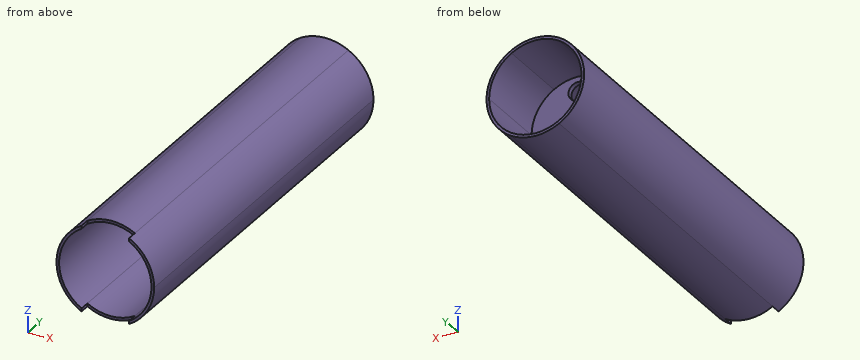
```python
from build123d import *

# Parameters (mm, degrees)
SHELL_DEPTH        = 150
SKETCH8_R          = 17.5
SKETCH8_R_2        = 3.5
SKETCH8_R_3        = 6.5
RODALIGNER_DEPTH   = 1
CUT_EXTRUDE1_DEPTH = 4


with BuildPart() as part:
    # Sketch1 → Shell (new body)
    with BuildSketch(Plane(origin=(0, 0, 0), x_dir=(1, 0, 0), z_dir=(0, 1, 0))):
        with BuildLine():
            ThreePointArc((-9.013878189, -15), (-17.5, 0), (-9.013878189, 15))
            Line((-9.013878189, 15), (-9.013878189, 16.155494421))
            ThreePointArc((-9.013878189, 16.155494421), (-18.5, 0), (-9.013878189, -16.155494421))
            Line((-9.013878189, -16.155494421), (-9.013878189, -15))
        make_face()
        with BuildLine():
            ThreePointArc((9.013878189, -15), (0, -17.5), (-9.013878189, -15))
            Line((-9.013878189, -15), (-9.013878189, -16.155494421))
            ThreePointArc((-9.013878189, -16.155494421), (0, -18.5), (9.013878189, -16.155494421))
            Line((9.013878189, -16.155494421), (9.013878189, -15))
        make_face()
        with BuildLine():
            Line((-9.013878189, 16.155494421), (-9.013878189, 15))
            ThreePointArc((-9.013878189, 15), (0, 17.5), (9.013878189, 15))
            Line((9.013878189, 15), (9.013878189, 16.155494421))
            ThreePointArc((9.013878189, 16.155494421), (0, 18.5), (-9.013878189, 16.155494421))
        make_face()
        with BuildLine():
            Line((9.013878189, 16.155494421), (9.013878189, 15))
            ThreePointArc((9.013878189, 15), (15.231429157, 8.617050879), (17.5, 0))
            ThreePointArc((17.5, 0), (15.231429157, -8.617050879), (9.013878189, -15))
            Line((9.013878189, -15), (9.013878189, -16.155494421))
            ThreePointArc((9.013878189, -16.155494421), (15.953161857, -9.367316945), (18.5, 0))
            ThreePointArc((18.5, 0), (15.953161857, 9.367316945), (9.013878189, 16.155494421))
        make_face()
    extrude(amount=SHELL_DEPTH)

    # Sketch8 → RodAligner (add, symmetric)
    with BuildSketch(Plane(origin=(0, 120, 0), x_dir=(1, 0, 0), z_dir=(0, 1, 0))):
        Circle(SKETCH8_R)
        with Locations((0, -12)):
            Circle(SKETCH8_R_2, mode=Mode.SUBTRACT)
        Circle(SKETCH8_R_3, mode=Mode.SUBTRACT)
    extrude(amount=RODALIGNER_DEPTH, both=True)

    # Sketch1_7 → Cut-Extrude1 (cut)
    with BuildSketch(Plane(origin=(0, 0, 0), x_dir=(1, 0, 0), z_dir=(0, 1, 0))):
        with BuildLine():
            Line((-9.013878189, 16.155494421), (-9.013878189, 15))
            ThreePointArc((-9.013878189, 15), (0, 17.5), (9.013878189, 15))
            Line((9.013878189, 15), (9.013878189, 16.155494421))
            ThreePointArc((9.013878189, 16.155494421), (0, 18.5), (-9.013878189, 16.155494421))
        make_face()
        with BuildLine():
            ThreePointArc((9.013878189, -15), (0, -17.5), (-9.013878189, -15))
            Line((-9.013878189, -15), (-9.013878189, -16.155494421))
            ThreePointArc((-9.013878189, -16.155494421), (0, -18.5), (9.013878189, -16.155494421))
            Line((9.013878189, -16.155494421), (9.013878189, -15))
        make_face()
    extrude(amount=CUT_EXTRUDE1_DEPTH, mode=Mode.SUBTRACT)


solid = part.part
```
Can you work these out from the model? Positions are in its coordinate system, mm. Coordinates: 2 decimals unless noted, no trailing zeros. Loops run counter-clockwise (first coordinate to the right, second up) from the corner with the lowest first, then second, coordinate; pieces in that order, holes last. Notation, with made-up numbers: (31.5, 14) -> (65.5, 14) arc R32 ccw to (65.5, 52) -> close; hole circle Ø11 at (-22, 6). An arc over 180 degrees is marked (long way). Put each result on its own line as item: value. Start each with the question number.
Q1. I want a section at A-A (x = 0). Write out the boundary of the cut face in (y, z), plus the area to 3 significant figures.
Q2. I want a section at C-C (z = 12). Write out the boundary of the cut face in (x, y).
Q3. I want a section at B-B (y = 10). Write out the boundary of the cut face in (x, z), plus the area to 3 significant figures.
Q4. If I drill on line 1 (Z direction, x = 0.5, y = 38); line 2 (Y direction, x = 9, z = -0.5); line 3 (X direction, y = 33, z = 9), over which ranges is the centre line in solid material (lowest first)? Write a range as [from, to].
Q5. I want a section at D-D (x = -16). Write out the boundary of the cut face in (y, z).
Q6. I'm going to push flat-ended pins straight in: P1, Ø17.5, axis at x = 0.5, z = 3, coming from the +Y side; P2, Ø1.1, axis at x = 1, z = -16.5, coming from the -Y side; P3, Ø8, axis at y = 132.5, z = -14, coming from the +X side; P4, Ø12, axis at x = -12, z = 3.5, coming from the +Y side. Where does each tip first touch, or does it pass through?
Taken from the geometry:
1. outline: (4, -18.5) -> (150, -18.5) -> (150, -17.5) -> (121, -17.5) -> (121, -6.5) -> (119, -6.5) -> (119, -17.5) -> (4, -17.5) -> close; (4, 17.5) -> (119, 17.5) -> (119, 15.5) -> (121, 15.5) -> (121, 17.5) -> (150, 17.5) -> (150, 18.5) -> (4, 18.5) -> close; (119, 6.5) -> (121, 6.5) -> (121, 8.5) -> (119, 8.5) -> close
1. area: 322 mm2
2. outline: (-14.08, 0) -> (-12.74, 0) -> (-12.74, 119) -> (-3.5, 119) -> (-3.5, 121) -> (-12.74, 121) -> (-12.74, 150) -> (-14.08, 150) -> close; (3.5, 119) -> (12.74, 119) -> (12.74, 0) -> (14.08, 0) -> (14.08, 150) -> (12.74, 150) -> (12.74, 121) -> (3.5, 121) -> close
3. outline: circle Ø37 at (0, 0); hole circle Ø35 at (0, 0)
3. area: 113 mm2
4. line 1: z = [-18.49, -17.49], [17.49, 18.49]
4. line 2: y = [119, 121]
4. line 3: x = [-16.16, -15.01], [15.01, 16.16]
5. outline: (0, -9.29) -> (150, -9.29) -> (150, -7.09) -> (121, -7.09) -> (121, 7.09) -> (150, 7.09) -> (150, 9.29) -> (0, 9.29) -> (0, 7.09) -> (119, 7.09) -> (119, -7.09) -> (0, -7.09) -> close
6. P1: stops at y = 121
6. P2: stops at y = 119
6. P3: stops at x = 15.56
6. P4: stops at y = 150
